Design review of the part built by this model. Coordinates are the model's own, in mm. Face numbers are marked on the shaded views. Round coordinates to 2 decimals unless told otherwise and drop trailing zeros. Order: outer loops, then holes, each group sorted by start corner. A loop starts at its lowest first (then second) coordinate and runs counter-clockwise, first axis right, second up. Notation, with made-up numbers: M -38,76 L 5,76 A17 ccw 5,92 Z; hole C 32,68.25 d2. An arc over 180 degrees is marked long. Use a Markdown table: item, result. Add a question column.
(1) Take a section at A-A (z = 0). Write out the cut boundary in (x, y), then the cut area to 3 significant figures.
(2) To check wall thickness, follow probe 1 along Z at (x, y) = (0.25, -9.5); probe 2 along Y at (x, z) = (3, -3); probe 3 along Y at (x, z) = (-4.5, -3.75). State the ranges of each line that lie inside material, in increasing order. Write a range as from..to.
(3) Take a section at C-C (y = -11.5). Write out the cut boundary in (x, z), then the cut area to 3 significant figures.
(4) For pin 1 (4 mm diameter, centred on x = 5.5, y = -24, fed in from -Z); pin 2 (3 mm diameter, centred on x = -1, y = -12.5, fed in from +Z); pin 3 (7 mm diameter, centred on x = 1, z = 0.5, fed in from -Y), all flat-tipped, find the tip position at first contact; note any pin that passes through.
(5) Take a section at B-B (x = 0). Write out the cut boundary in (y, z).
(6) The part is to be moulded in two halves that separate along X. For the marked faces 1, 2 and 3, say which applies: released by +X, released by -X, zero draft, split by the parting line, or undercut.
```python
from build123d import *

# Parameters (mm, degrees)
F2_R     = 1
F3_R     = 0.25
F4_R     = 5
F5_DEPTH = 39


with BuildPart() as f1:
    # F0 (on Top) → F1 (revolve)
    with BuildSketch(Plane.XY):
        Polygon((-6.34, -37.18), (0, -37.18), (0, 9.81), (-5.73, 9.81), (-5.73, 1.94), (-7.39, 1.94), (-7.39, 0), (-6.34, 0), align=None)
    revolve(axis=Axis((0, -13.32371, 0), (0, 1, 0)))

    # F2
    f2_edges = [f1.edges().sort_by_distance(p)[0] for p in [
        (5.73, 9.81, 0),
    ]]
    fillet(f2_edges, radius=F2_R)

    # F3
    f3_edges = [f1.edges().sort_by_distance(p)[0] for p in [
        (7.39, 1.94, 0),
        (7.39, 0, 0),
        (-7.39, 0.97, 0),
    ]]
    fillet(f3_edges, radius=F3_R)

    # F4 (on face) → F5 (cut)
    with BuildSketch(Plane.XZ.offset(37.18)):
        Circle(F4_R)
    extrude(amount=-F5_DEPTH, mode=Mode.SUBTRACT)


solid = f1.part
```
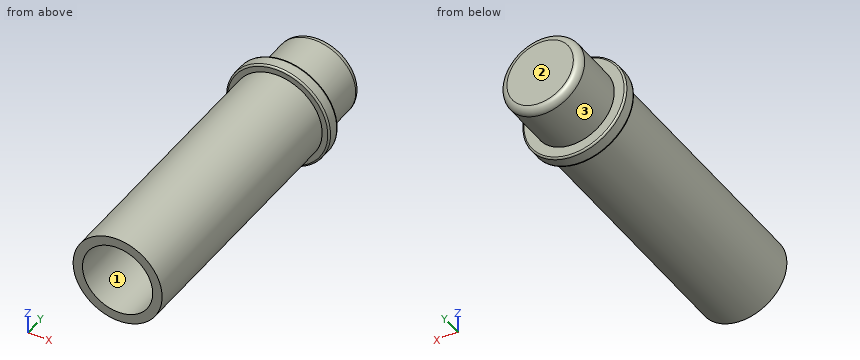
Verdict:
| question | item | result |
|---|---|---|
| 1 | outline | M -7.39,0.25 A0.25 ccw -7.14,0 L -6.34,0 L -6.34,-37.18 L -5,-37.18 L -5,1.82 L 5,1.82 L 5,-37.18 L 6.34,-37.18 L 6.34,0 L 7.14,0 A0.25 ccw 7.39,0.25 L 7.39,1.69 A0.25 ccw 7.14,1.94 L 5.73,1.94 L 5.73,8.81 A1 ccw 4.73,9.81 L -4.73,9.81 A1 ccw -5.73,8.81 L -5.73,1.94 L -7.14,1.94 A0.25 ccw -7.39,1.69 Z |
| 1 | area | 200 mm^2 |
| 2 | probe 1 | z = -6.34..-4.99, 4.99..6.34 |
| 2 | probe 2 | y = 1.82..9.81 |
| 2 | probe 3 | y = -37.18..1.94 |
| 3 | outline | C 0,0 d12.68; hole C 0,0 d10 |
| 3 | area | 47.7 mm^2 |
| 4 | pin 1 | stops at z = -5.29 |
| 4 | pin 2 | stops at z = 6.34 |
| 4 | pin 3 | stops at y = 1.82 |
| 5 | outline | M -37.18,-6.34 L 0,-6.34 L 0,-7.14 A0.25 ccw 0.25,-7.39 L 1.69,-7.39 A0.25 ccw 1.94,-7.14 L 1.94,-5.73 L 8.81,-5.73 A1 ccw 9.81,-4.73 L 9.81,4.73 A1 ccw 8.81,5.73 L 1.94,5.73 L 1.94,7.14 A0.25 ccw 1.69,7.39 L 0.25,7.39 A0.25 ccw 0,7.14 L 0,6.34 L -37.18,6.34 L -37.18,5 L 1.82,5 L 1.82,-5 L -37.18,-5 Z |
| 6 | face 1 | undercut |
| 6 | face 2 | zero draft |
| 6 | face 3 | split by the parting line |
